from build123d import *

# Parameters (mm, degrees)
BOSS_EXTRUDE1_DEPTH = 25
SKETCH3_R           = 3.5
SKETCH3_R_2         = 3
CUT_EXTRUDE1_DEPTH  = 30
SKETCH5_R           = 12.25
CUT_EXTRUDE3_DEPTH  = 299.5
SKETCH8_R           = 20
CUT_EXTRUDE6_DEPTH  = 299.5
SKETCH7_R           = 28.5
CUT_EXTRUDE5_DEPTH  = 12.55
SKETCH9_R           = 21
CUT_EXTRUDE7_DEPTH  = 12
SKETCH18_R          = 3.500000003
CUT_EXTRUDE11_DEPTH = 70
SKETCH25_R          = 4.5
CUT_EXTRUDE18_DEPTH = 15
CUT_EXTRUDE19_START = -15
SKETCH26_R          = 4.5
CUT_EXTRUDE19_DEPTH = 15
CUT_EXTRUDE22_DEPTH = 2
CUT_EXTRUDE23_START = -2
CUT_EXTRUDE23_DEPTH = 2


with BuildPart() as part:
    # Sketch2 → Boss-Extrude1 (new body)
    with BuildSketch(Plane.XY):
        Polygon((-180.451457822, 33.745151522), (-172.941457822, 33.745151522), (-172.941457822, 93.745151522), (-268.451457822, 93.745151522), (-268.451457822, 33.745151522), align=None)
    extrude(amount=BOSS_EXTRUDE1_DEPTH)

    # Sketch3 → Cut-Extrude1 (cut)
    with BuildSketch(Plane(origin=(-254.526795804, 25.613966889, 25), x_dir=(1, 0, 0), z_dir=(0, 0, 1))):
        with Locations((-7.924662018, 60.131184633)):
            Circle(SKETCH3_R)
        with Locations((69.075337951, 60.131184633)):
            Circle(SKETCH3_R_2)
        with Locations((69.075337951, 16.131184633)):
            Circle(SKETCH3_R)
        with Locations((-7.924662018, 16.131184633)):
            Circle(SKETCH3_R)
    extrude(amount=-CUT_EXTRUDE1_DEPTH, mode=Mode.SUBTRACT)

    # Sketch5 → Cut-Extrude3 (cut)
    with BuildSketch(Plane(origin=(-254.526795796, 218.819962105, 46.890114798), x_dir=(0, 0, 1), z_dir=(0, 1, 0))):
        with Locations((-21.890114798, 51.081437247)):
            Circle(SKETCH5_R)
    extrude(amount=-CUT_EXTRUDE3_DEPTH, mode=Mode.SUBTRACT)

    # Sketch8 → Cut-Extrude6 (cut)
    with BuildSketch(Plane(origin=(-254.526795804, 25.613966889, 25), x_dir=(1, 0, 0), z_dir=(0, 0, 1))):
        with Locations((16.121848571, 37.941765268)):
            Circle(SKETCH8_R)
    extrude(amount=-CUT_EXTRUDE6_DEPTH, mode=Mode.SUBTRACT)

    # Sketch7 → Cut-Extrude5 (cut)
    with BuildSketch(Plane(origin=(-254.526795804, 25.613966889, 25), x_dir=(1, 0, 0), z_dir=(0, 0, 1))):
        with Locations((16.121848571, 37.941765268)):
            Circle(SKETCH7_R)
    extrude(amount=-CUT_EXTRUDE5_DEPTH, mode=Mode.SUBTRACT)

    # Sketch9 → Cut-Extrude7 (cut)
    with BuildSketch(Plane.XY.offset(12.45)):
        with Locations((-238.404947233, 63.555732157)):
            Circle(SKETCH9_R)
    extrude(amount=-CUT_EXTRUDE7_DEPTH, mode=Mode.SUBTRACT)

    # Sketch18 → Cut-Extrude11 (cut)
    with BuildSketch(Plane(origin=(-155.753430747, 103.745151522, -13.013772077), x_dir=(0, 0, 1), z_dir=(0, 1, 0))):
        with Locations((21.263772077, -72.191927802)):
            Circle(SKETCH18_R)
        with Locations((21.263772077, -23.191927802)):
            Circle(SKETCH18_R)
    extrude(amount=-CUT_EXTRUDE11_DEPTH, mode=Mode.SUBTRACT)

    # Sketch25 → Cut-Extrude18 (cut)
    with BuildSketch(Plane(origin=(-254.526795796, 93.745151522, 46.890114798), x_dir=(0, 0, 1), z_dir=(0, 1, 0))):
        with Locations((-21.890114798, 0.672048442)):
            Circle(SKETCH25_R)
    extrude(amount=-CUT_EXTRUDE18_DEPTH, mode=Mode.SUBTRACT)

    # Sketch26 → Cut-Extrude19 (cut)
    with BuildSketch(Plane(origin=(-254.526795796, 33.745151522, 3.109885202), x_dir=(0, 0, -1), z_dir=(0, -1, 0)).offset(CUT_EXTRUDE19_START)):
        with Locations((-21.890114798, 0.672048442)):
            Circle(SKETCH26_R)
    extrude(amount=CUT_EXTRUDE19_DEPTH, mode=Mode.SUBTRACT)

    # Sketch29 → Cut-Extrude22 (cut)
    with BuildSketch(Plane(origin=(-217.163449612, 32.745151522, 13.13747962), x_dir=(-1, 0, 0), z_dir=(0, -1, 0))):
        with BuildLine():
            ThreePointArc((36.691297742, -16.86252038), (41.691297742, -11.86252038), (36.691297742, -6.86252038))
            ThreePointArc((36.691297742, -6.86252038), (31.691297742, -11.86252038), (36.691297742, -16.86252038))
        make_face()
    extrude(amount=-CUT_EXTRUDE22_DEPTH, mode=Mode.SUBTRACT)

    # Sketch30 → Cut-Extrude23 (cut)
    with BuildSketch(Plane(origin=(-217.163449612, 94.745151522, 36.86252038), x_dir=(-1, 0, 0), z_dir=(0, 1, 0)).offset(CUT_EXTRUDE23_START)):
        with BuildLine():
            ThreePointArc((36.691297742, -16.86252038), (41.691297742, -11.86252038), (36.691297742, -6.86252038))
            ThreePointArc((36.691297742, -6.86252038), (31.691297742, -11.86252038), (36.691297742, -16.86252038))
        make_face()
    extrude(amount=CUT_EXTRUDE23_DEPTH, mode=Mode.SUBTRACT)


solid = part.part
Input: part model. Units: mm. Frame: model coordinates. A direction names the side the tool comes from. Round coordinates to 2 decimals unless told otherwise and drop trailing zeros. Order: outer loops, then holes, each group sorted by start corner. A loop starts at its lowest first (then second) coordinate and runs counter-clockwise, first axis right, second up.
1. Cut plane B-B, the plane y = 57. Output: boundary loops of the cut face in (x, z).
The answers:
outline: (-268.45, 0) - (-257.3, 0) - (-257.3, 0.45) - (-258.36, 0.45) - (-258.36, 12.45) - (-266.14, 12.45) - (-266.14, 25) - (-268.45, 25) - close; (-219.51, 0) - (-172.94, 0) - (-172.94, 25) - (-191.2, 25) arc R12.25 cw to (-210.67, 15.11) - (-210.67, 12.45) - (-218.45, 12.45) - (-218.45, 0.45) - (-219.51, 0.45) - close; hole circle Ø7 at (-178.95, 8.25)
2. Material intervals for line 1 (X direction, y = 41.5, z = 15); line 2 (X direction, y = 88, z = 20); line 3 (X direction, y = 76.5, z = 14), sorted ascending.
The answers:
line 1: x = -268.45 to -265.94, -258.96 to -256.45, -220.36 to -210.52, -196.37 to -188.94, -181.96 to -172.94
line 2: x = -268.45 to -265.13, -259.77 to -253.06, -223.75 to -214.63, -192.26 to -187.43, -183.47 to -172.94
line 3: x = -268.45 to -263.8, -213.01 to -208.84, -198.05 to -172.94
3. Cut plane A-A, the plane z = 8.25. Output: boundary loops of the cut face in (x, y).
The answers:
outline: (-268.45, 33.75) - (-231.45, 33.75) - (-231.45, 43.74) arc R21 cw (long way) to (-231.45, 83.37) - (-231.45, 93.75) - (-268.45, 93.75) - close; (-224.45, 33.75) - (-182.45, 33.75) - (-182.45, 39.95) arc R3.5 cw (long way) to (-182.45, 43.54) - (-182.45, 93.75) - (-224.45, 93.75) - (-224.45, 79.24) arc R21 cw to (-224.45, 47.87) - close; (-175.45, 33.75) - (-172.94, 33.75) - (-172.94, 93.75) - (-175.45, 93.75) - close; hole circle Ø7 at (-262.45, 41.75); hole circle Ø7 at (-262.45, 85.75); hole circle Ø6 at (-185.45, 85.75)
4. Set-up query: faces 1 (the face through (-259.385, 64.479, 6.534)), 2 (the face through (-199.003, 64.165, 13.584)), 3 (the face through (-253.96, 34.24, 20)). Return all of +Z, -Z, +X, -X, +Y, -Y with unobstructed straight access to the full face (end or side cutting, diameter ignored); none if empty.
The answers:
face 1: +Z
face 2: +Z, +Y, -Y
face 3: +Z, -Y
5. Cut plane D-D, the plane x = -225.5. Output: boundary loops of the cut face in (y, z).
The answers:
outline: (33.75, 0) - (48.28, 0) - (48.28, 0.45) - (46.99, 0.45) - (46.99, 5.75) - (33.75, 5.75) - close; (33.75, 10.75) - (46.99, 10.75) - (46.99, 12.45) - (38.14, 12.45) - (38.14, 25) - (33.75, 25) - close; (78.84, 0) - (93.75, 0) - (93.75, 5.75) - (80.12, 5.75) - (80.12, 0.45) - (78.84, 0.45) - close; (80.12, 10.75) - (93.75, 10.75) - (93.75, 25) - (88.97, 25) - (88.97, 12.45) - (80.12, 12.45) - close
6. Pin query (flat end, axial travel): P1, Ø12.5, axis at x = -239, y = 56, coming from the +Z side; P2, Ø1.5, axis at x = -218.5, y = 70, coming from the +Z side. Return the tip coordinate at first contact, or that it passes through.
The answers:
P1: passes through
P2: stops at z = 12.45
7. Cut plane C-C, the plane z = 22.5. State how many separate pieces and enclosed holes the cut face has, then the cut area to 3 significant figures.
The answers:
separate pieces: 4
enclosed holes: 4
area: 1,630 mm2
8. Mould query, pull axis Z, two halves, no side actions, for faces 4 (the face through (-253.74, 93.24, 20)), 5 (the face through (-259.22, 84.4, 12.68)), 6 (the face through (-224.475, 39.336, 7.794)). Classes: released by +Z, released by -Z, zero draft, split by the parting line, or undercut.
The answers:
face 4: released by +Z
face 5: zero draft
face 6: undercut
